```python
from build123d import *

# Parameters (mm, degrees)
F0_R     = 279.4
F1_DEPTH = 101.6
F2_R     = 12.7
F2_R_2   = 12.5
F3_DEPTH = 50.8


with BuildPart() as f1:
    # F0 (on Top) → F1 (new body)
    with BuildSketch(Plane.XY):
        with BuildLine():
            ThreePointArc((165.1, -285.961588), (285.961588, -165.1), (330.2, 0))
            ThreePointArc((330.2, 0), (316.035905, 95.673125), (274.758772, 183.138356))
            ThreePointArc((274.758772, 183.138356), (225.85856, 240.873309), (165.1, 285.961588))
            ThreePointArc((165.1, 285.961588), (-95.673125, 316.035905), (-295.981854, 146.378898))
            ThreePointArc((-295.981854, 146.378898), (-321.531685, 75.162596), (-330.2, 0))
            ThreePointArc((-330.2, 0), (-225.85856, -240.873309), (21.223083, -329.517254))
            ThreePointArc((21.223083, -329.517254), (95.673125, -316.035905), (165.1, -285.961588))
        make_face()
        Circle(F0_R, mode=Mode.SUBTRACT)
        with BuildLine():
            ThreePointArc((165.1, 285.961588), (225.85856, 240.873309), (274.758772, 183.138356))
            ThreePointArc((274.758772, 183.138356), (419.955029, 555.806639), (346.296428, 948.919871))
            ThreePointArc((346.296428, 948.919871), (343.096456, 900.151785), (327.593656, 853.80279))
            ThreePointArc((327.593656, 853.80279), (346.365994, 854.936106), (365.172292, 855.026849))
            Line((365.172292, 855.026849), (386.159106, 781.773906))
            ThreePointArc((386.159106, 781.773906), (330.519346, 792.374089), (274.106758, 787.298))
            ThreePointArc((274.106758, 787.298), (233.337853, 773.127606), (196.453349, 750.712498))
            ThreePointArc((196.453349, 750.712498), (183.140497, 739.629863), (170.813812, 727.459832))
            Line((170.813812, 727.459832), (159.193876, 746.42974))
            ThreePointArc((159.193876, 746.42974), (148.199724, 746.572871), (137.232142, 747.350049))
            ThreePointArc((137.232142, 747.350049), (210.182068, 520.220384), (165.1, 285.961588))
        make_face()
        with BuildLine():
            ThreePointArc((219.740654, 389.881855), (289.102738, 373.429577), (335.428058, 319.247098))
            Line((335.428058, 319.247098), (315.070275, 279.674231))
            ThreePointArc((315.070275, 279.674231), (278.207397, 339.338206), (208.315586, 345.151683))
            Line((208.315586, 345.151683), (219.740654, 389.881855))
        make_face(mode=Mode.SUBTRACT)
        with BuildLine():
            ThreePointArc((230.090316, 495.358171), (318.97663, 501.347432), (378.566059, 435.122451))
            Line((378.566059, 435.122451), (364.622182, 390.380044))
            ThreePointArc((364.622182, 390.380044), (308.575729, 448.660988), (227.861751, 443.851925))
            Line((227.861751, 443.851925), (230.090316, 495.358171))
        make_face(mode=Mode.SUBTRACT)
        with BuildLine():
            ThreePointArc((220.506904, 588.747772), (315.233937, 615.350933), (401.950913, 568.863247))
            Line((401.950913, 568.863247), (395.450001, 513.362684))
            ThreePointArc((395.450001, 513.362684), (315.191991, 550.934084), (228.323604, 533.417188))
            Line((228.323604, 533.417188), (220.506904, 588.747772))
        make_face(mode=Mode.SUBTRACT)
        with BuildLine():
            ThreePointArc((190.731506, 685.758289), (287.267753, 744.917108), (397.553807, 719.304627))
            Line((397.553807, 719.304627), (403.311044, 656.066156))
            ThreePointArc((403.311044, 656.066156), (302.181037, 674.537443), (211.661495, 625.806762))
            Line((211.661495, 625.806762), (190.731506, 685.758289))
        make_face(mode=Mode.SUBTRACT)
        with BuildLine():
            ThreePointArc((578.608057, -492.521545), (345.433034, -442.133203), (165.1, -285.961588))
            ThreePointArc((165.1, -285.961588), (95.673125, -316.035905), (21.223083, -329.517254))
            ThreePointArc((21.223083, -329.517254), (271.365154, -641.595043), (648.6405, -774.36144))
            ThreePointArc((648.6405, -774.36144), (608.006084, -747.206139), (575.618078, -710.605824))
            ThreePointArc((575.618078, -710.605824), (567.21339, -727.429803), (557.888826, -743.761906))
            Line((557.888826, -743.761906), (483.95651, -725.310549))
            ThreePointArc((483.95651, -725.310549), (520.956418, -682.425195), (544.76669, -631.032416))
            ThreePointArc((544.76669, -631.032416), (552.879221, -588.640311), (551.90942, -545.489839))
            ThreePointArc((551.90942, -545.489839), (548.968002, -528.419254), (544.591788, -511.659017))
            Line((544.591788, -511.659017), (566.830179, -511.080811))
            ThreePointArc((566.830179, -511.080811), (572.45121, -501.631161), (578.608057, -492.521545))
        make_face()
        with BuildLine():
            ThreePointArc((227.777264, -385.241916), (178.848131, -437.085104), (108.762068, -450.112768))
            Line((108.762068, -450.112768), (84.669851, -412.695977))
            ThreePointArc((84.669851, -412.695977), (154.771808, -410.603776), (194.752332, -352.982431))
            Line((194.752332, -352.982431), (227.777264, -385.241916))
        make_face(mode=Mode.SUBTRACT)
        with BuildLine():
            ThreePointArc((313.947602, -446.943144), (274.691297, -526.915581), (187.544067, -545.40905))
            Line((187.544067, -545.40905), (155.767944, -510.962094))
            ThreePointArc((155.767944, -510.962094), (234.263949, -491.564914), (270.456167, -419.260027))
            Line((270.456167, -419.260027), (313.947602, -446.943144))
        make_face(mode=Mode.SUBTRACT)
        with BuildLine():
            ThreePointArc((399.617075, -485.338467), (375.292572, -580.676064), (291.674567, -632.531325))
            Line((291.674567, -632.531325), (246.860125, -599.151088))
            ThreePointArc((246.860125, -599.151088), (319.526917, -548.431313), (347.791033, -464.442635))
            Line((347.791033, -464.442635), (399.617075, -485.338467))
        make_face(mode=Mode.SUBTRACT)
        with BuildLine():
            ThreePointArc((498.518346, -508.057474), (501.483263, -621.239726), (424.159177, -703.94401))
            Line((424.159177, -703.94401), (366.514436, -677.310688))
            ThreePointArc((366.514436, -677.310688), (433.076043, -598.965176), (436.133807, -496.207613))
            Line((436.133807, -496.207613), (498.518346, -508.057474))
        make_face(mode=Mode.SUBTRACT)
        with BuildLine():
            ThreePointArc((327.593656, 853.80279), (343.096456, 900.151785), (346.296428, 948.919871))
            ThreePointArc((346.296428, 948.919871), (23.952295, 1074.045306), (137.232142, 747.350049))
            ThreePointArc((137.232142, 747.350049), (148.199724, 746.572871), (159.193876, 746.42974))
            Line((159.193876, 746.42974), (140.616896, 776.757238))
            ThreePointArc((140.616896, 776.757238), (228.227479, 829.544451), (327.593656, 853.80279))
        make_face()
        Polygon((75.530644, 936.905829), (115.853144, 1006.746447), (196.498144, 1006.746447), (236.820644, 936.905829), (196.498144, 867.06521), (115.853144, 867.06521), align=None, mode=Mode.SUBTRACT)
        with BuildLine():
            ThreePointArc((648.6405, -774.36144), (918.174372, -557.765949), (578.608057, -492.521545))
            ThreePointArc((578.608057, -492.521545), (572.45121, -501.631161), (566.830179, -511.080811))
            Line((566.830179, -511.080811), (602.383053, -510.156423))
            ThreePointArc((602.383053, -510.156423), (604.292829, -612.42302), (575.618078, -710.605824))
            ThreePointArc((575.618078, -710.605824), (608.006084, -747.206139), (648.6405, -774.36144))
        make_face()
        Polygon((773.618927, -533.864371), (813.941427, -603.704989), (773.618927, -673.545608), (692.973927, -673.545608), (652.651427, -603.704989), (692.973927, -533.864371), align=None, mode=Mode.SUBTRACT)
        with BuildLine():
            ThreePointArc((-330.2, 0), (-321.531685, 75.162596), (-295.981854, 146.378898))
            ThreePointArc((-295.981854, 146.378898), (-691.320184, 85.788404), (-994.936929, -174.558431))
            ThreePointArc((-994.936929, -174.558431), (-951.102541, -152.945645), (-903.211734, -143.196967))
            ThreePointArc((-903.211734, -143.196967), (-913.579384, -127.506303), (-923.061118, -111.264943))
            Line((-923.061118, -111.264943), (-870.115616, -56.463358))
            ThreePointArc((-870.115616, -56.463358), (-851.475764, -109.948895), (-818.873448, -156.265585))
            ThreePointArc((-818.873448, -156.265585), (-786.217073, -184.487295), (-748.362768, -205.222658))
            ThreePointArc((-748.362768, -205.222658), (-732.108499, -211.210609), (-715.405601, -215.800815))
            Line((-715.405601, -215.800815), (-726.024055, -235.34893))
            ThreePointArc((-726.024055, -235.34893), (-720.650934, -244.94171), (-715.840199, -254.828503))
            ThreePointArc((-715.840199, -254.828503), (-555.615102, -78.087181), (-330.2, 0))
        make_face()
        with BuildLine():
            ThreePointArc((-689.249852, -177.700815), (-788.751016, -123.677382), (-821.712984, -15.360618))
            Line((-821.712984, -15.360618), (-769.82548, 21.244532))
            ThreePointArc((-769.82548, 21.244532), (-735.25708, -75.572267), (-647.795302, -129.59915))
            Line((-647.795302, -129.59915), (-689.249852, -177.700815))
        make_face(mode=Mode.SUBTRACT)
        with BuildLine():
            Line((-576.114637, -68.974553), (-620.12398, -103.409305))
            ThreePointArc((-620.12398, -103.409305), (-690.526509, -34.674869), (-693.62548, 63.668078))
            Line((-693.62548, 63.668078), (-642.310126, 85.788404))
            ThreePointArc((-642.310126, 85.788404), (-634.718908, -2.502771), (-576.114637, -68.974553))
        make_face(mode=Mode.SUBTRACT)
        with BuildLine():
            Line((-498.317918, -24.591898), (-544.037918, -48.415027))
            ThreePointArc((-544.037918, -48.415027), (-593.667927, 25.568149), (-566.110126, 110.286599))
            Line((-566.110126, 110.286599), (-520.390126, 120.582051))
            ThreePointArc((-520.390126, 120.582051), (-542.839678, 42.903926), (-498.317918, -24.591898))
        make_face(mode=Mode.SUBTRACT)
        with BuildLine():
            ThreePointArc((-447.517918, -4.639939), (-467.950869, 63.655527), (-444.190126, 130.86567))
            Line((-444.190126, 130.86567), (-399.740126, 133.021747))
            ThreePointArc((-399.740126, 133.021747), (-432.979205, 71.26557), (-403.067918, 7.830748))
            Line((-403.067918, 7.830748), (-447.517918, -4.639939))
        make_face(mode=Mode.SUBTRACT)
        with BuildLine():
            ThreePointArc((-903.211734, -143.196967), (-951.102541, -152.945645), (-994.936929, -174.558431))
            ThreePointArc((-994.936929, -174.558431), (-942.126667, -516.279357), (-715.840199, -254.828503))
            ThreePointArc((-715.840199, -254.828503), (-720.650934, -244.94171), (-726.024055, -235.34893))
            Line((-726.024055, -235.34893), (-742.999948, -266.600815))
            ThreePointArc((-742.999948, -266.600815), (-832.520308, -217.121431), (-903.211734, -143.196967))
        make_face()
        Polygon((-849.14957, -263.360221), (-808.82707, -333.200839), (-849.14957, -403.041458), (-929.79457, -403.041458), (-970.11707, -333.200839), (-929.79457, -263.360221), align=None, mode=Mode.SUBTRACT)
    extrude(amount=F1_DEPTH)

    # F2 (on face) → F3 (cut)
    with BuildSketch(Plane.XY.offset(101.6)):
        with Locations((138.178983, -380.014748)):
            Circle(F2_R)
        with Locations((260.012934, 309.673884)):
            Circle(F2_R)
        with Locations((-398.191917, 70.340864)):
            Circle(F2_R)
        with Locations((866.295139, -604.290373)):
            Circle(F2_R_2)
        with Locations((90.183245, 1052.378784)):
            Circle(F2_R_2)
        with Locations((-956.478384, -448.088411)):
            Circle(F2_R_2)
    extrude(amount=-F3_DEPTH, mode=Mode.SUBTRACT)


solid = f1.part
```
CAD build for the part. Positions are in the model's coordinates, mm. Coordinates: 2 decimals unless noted, no trailing zeros. Order: outer loops, then holes, each group sorted by start corner. A loop starts at its lowest first (then second) coordinate and runs counter-clockwise, first axis right, second up. Notation, with made-up numbers: (13.5, -3.5) -> (41.5, -3.5) arc R26 cw to (41.5, 22.5) -> close; hole circle Ø9 at (-27.75, -3). An arc over 180 degrees is marked (long way). Use one line per item in the form item = value. Start each with the question number.
1) Band-saw the part on A-A on x = -250. Give the cut face in (y, z).
2) Band-saw the part on B-B on z = 83. State how many separate pieces and enclosed holes the cut face has, then the cut area to 3 significant figures.
3) Pull direction X, two halves, no side cores. Call faces 1 (the cylindrical face through (419.405, 550.161, 50.089)), 2 (the flat face through (216.377, 972.315, 50.089)), 3 (the cylindrical face through (28.4, 1078.2, 50.1)), 4 (the cylindrical face through (303.63, 674.76, 50.09)): +X half, -X half, draft (parallel to the pull), parting line (faces both ways), or undercut.
4) Drop flat-ended pins along their axis: pin 1 (20.5 mm diameter, centred on x = 138.18, y = -380.01, fed in from +Z); pin 2 (2 mm diameter, centred on x = -823.5, z = 57, fed in from -Y); pin 3 (8 mm diameter, centred on x = 307, z = 81, fed in from -Y). Give the stop position or say it passes through.
5) Drill centre lines: L1, parallel to Y at x = -783, z = 20; L2, parallel to X at y = -619.5, z = 75; L3, parallel to X at y = -654, z = 88. Where is each one in solid material? Low to high. Write a range as [from, to].
Entries:
q1.outline = (-215.71, 0) -> (-124.76, 0) -> (-124.76, 101.6) -> (-215.71, 101.6) -> close; (124.76, 0) -> (215.71, 0) -> (215.71, 101.6) -> (124.76, 101.6) -> close
q2.separate_pieces = 1
q2.enclosed_holes = 25
q2.area = 592,000 mm2
q3.face_1 = +X half
q3.face_2 = undercut
q3.face_3 = parting line
q3.face_4 = undercut
q4.pin_1 = 50.8
q4.pin_2 = -512.28
q4.pin_3 = -667.8
q5.L1 = [-491.17, -248.83], [-186.68, -130.32], [11.95, 35.42]
q5.L2 = [241.82, 274.18], [330.11, 423.41], [502.13, 547.9], [603.27, 661.77], [804.82, 923.14]
q5.L3 = [289.43, 396.98], [484.12, 536.26], [596.07, 681.69], [784.9, 917.04]
